from build123d import *

# Parameters (mm, degrees)
BOSS_EXTRUDE2_DEPTH = 5
BOSS_EXTRUDE3_DEPTH = 20.3
BOSS_EXTRUDE4_DEPTH = 5


with BuildPart() as part:
    # Sketch3 → Boss-Extrude2 (new body)
    with BuildSketch(Plane(origin=(0, 0, 0), x_dir=(1, 0, 0), z_dir=(0, 1, 0))):
        Polygon((-54.461524227, -2.229452052), (-41.811524227, -24.139894768), (0, -24.139894768), (0, 29.213923621), (0, 53.936652846), (-65.166780007, 16.312594867), align=None)
    extrude(amount=BOSS_EXTRUDE2_DEPTH)

    # Sketch4 → Boss-Extrude3 (add)
    with BuildSketch(Plane(origin=(0, 5, 0), x_dir=(1, 0, 0), z_dir=(0, 1, 0))):
        Polygon((-51.961524227, -6.559579071), (0, 23.440420929), (0, 29.213923621), (0, 53.936652846), (-65.166780007, 16.312594867), (-54.461524227, -2.229452052), align=None)
    extrude(amount=BOSS_EXTRUDE3_DEPTH)

    # Sketch5 → Boss-Extrude4 (add)
    with BuildSketch(Plane(origin=(0, 25.3, 0), x_dir=(1, 0, 0), z_dir=(0, 1, 0))):
        Polygon((-65.166780007, 16.312594867), (-41.811524227, -24.139894768), (0, -24.139894768), (0, 53.936652846), align=None)
    extrude(amount=BOSS_EXTRUDE4_DEPTH)


solid = part.part
Geometry check sheet. Reference: the model listing, model coordinates, mm. A direction names the side the tool comes from. Coordinates: 2 decimals unless noted, no trailing zeros. Order: outer loops, then holes, each group sorted by start corner. A loop starts at its lowest first (then second) coordinate and runs counter-clockwise, first axis right, second up. Notation, with made-up numbers: (48.25, 75.25) - (71.25, 75.25) arc R27 ccw to (71.25, 101.25) - close; hole circle Ø6 at (20, 10.5). An arc over 180 degrees is marked (long way). Answer in a Markdown table with one row per item. Add a question column.
1) Gauge pin test, flat ends, axial feed: P1, Ø2, axis at x = -28, y = 6.5, coming from the -Z side; P2, Ø3, axis at y = 11.5, z = -34, coming from the -X side; P3, Ø4, axis at x = -37.5, y = 12, coming from the +Z side. Record the tip position at first contact, or that the pin passes through.
2) Cross-section at A-A, the plane z = 13. Record the cut outline in (x, y), then the cut area to 3 significant figures.
3) Cross-section at B-B, the plane x = -31. Record the cut outline in (y, z).
4) Cross-section at C-C, the plane y = 14.5. Record the cut outline in (x, z), then the cut area to 3 significant figures.
5) Material ranges on line 1 along Y through (x, z) = (-5, -13); line 2 along Z through (x, y) = (-38, 19); line 3 along X through (y, z) = (11, -29.5), recorded low to high. Write a range as [from, to].
6) Set-up check for faces 1 (the flat face through (-21, 25.3, 5)), 2 (the flat face through (-26, 0, -7)): record each of +Z, -Z, +X, -X, +Y, -Y from which the full face is reachable in a straight line by a thin tool's end or side.
7) Release check for a two-part mould opening along Y. For faces 3 (the flat face through (-26, 30.3, -7)), 4 (the flat face through (-21, 5, 5)), 5 (the flat face through (-26.344, 15.008, -8.23)), 6 (the flat face through (-21, 28, 24.14)) record: +Y half, -Y half, draft (parallel to the pull), parting line (faces both ways), or undercut.
8) Cross-section at D-D, the plane z = -6.5. Record the cut outline in (x, y).
Check result:
| question | item | result |
|---|---|---|
| 1 | P1 | stops at z = -38.35 |
| 1 | P2 | stops at x = -37.13 |
| 1 | P3 | stops at z = -0.64 |
| 2 | outline | (-48.24, 0) - (0, 0) - (0, 5) - (-48.24, 5) - close; (-48.24, 25.3) - (0, 25.3) - (0, 30.3) - (-48.24, 30.3) - close |
| 2 | area | 482 mm² |
| 3 | outline | (0, -36.04) - (30.3, -36.04) - (30.3, 24.14) - (25.3, 24.14) - (25.3, -5.54) - (5, -5.54) - (5, 24.14) - (0, 24.14) - close |
| 4 | outline | (-65.17, -16.31) - (0, -53.94) - (0, -23.44) - (-51.96, 6.56) - close |
| 4 | area | 1,790 mm² |
| 5 | line 1 | y = [0, 5], [25.3, 30.3] |
| 5 | line 2 | z = [-32, -1.5] |
| 5 | line 3 | x = [-42.33, 0] |
| 6 | face 1 | +Z, +X |
| 6 | face 2 | +Z, -Z, +X, -X, -Y |
| 7 | face 3 | +Y half |
| 7 | face 4 | undercut |
| 7 | face 5 | undercut |
| 7 | face 6 | draft |
| 8 | outline | (-59.5, 0) - (0, 0) - (0, 5) - (-29.34, 5) - (-29.34, 25.3) - (0, 25.3) - (0, 30.3) - (-59.5, 30.3) - close |
